Verification items for the finished model (mm, model axes). Face numbers are marked on the shaded views. A direction names the side the tool comes from. Round coordinates to 2 decimals unless told otherwise and drop trailing zeros. Write each loop counter-clockwise with the first axis right and the second up, starting at its lowest first coordinate (ties: lowest second). Pieces come first, ordered by that corner, then holes. Notation, with made-up numbers: M 38.5,28.25 L 50.5,28.25 A23 cw 50.5,51.25 Z; hole C -18,22.5 d4. An arc over 180 degrees is marked long. Answer in a Markdown table with one row per item. Add a question column.
1. Sectioned sample at A-A on z = 0. Record the cut outline in (x, y), plus the area to 3 significant figures.
2. Go/stop test with flat-tipped pins: pin 1 Ø2 at (x, y) = (1, 3) entering from -Z; pin 2 Ø3 at (x, y) = (7, 1) entering from -Z; pin 3 Ø2 at (x, y) = (-6.5, 5) entering from -Z. Record where each tip stops, or that it passes through.
3. Material ranges on probe 1 along X at (y, z) = (3, 0); probe 2 along Z at (x, y) = (1, 1.6); probe 3 along Y at (x, z) = (7, 5.75), recorded low to high.
4. Sectioned sample at B-B on y = 0.9. Record the cut outline in (x, z), plus the area to 3 significant figures.
5. Set-up check for the marked faces 1 and 2: record each of +Z, -Z, +X, -X, +Y, -Y from which the full face is reachable in a straight line by a thin tool's end or side.
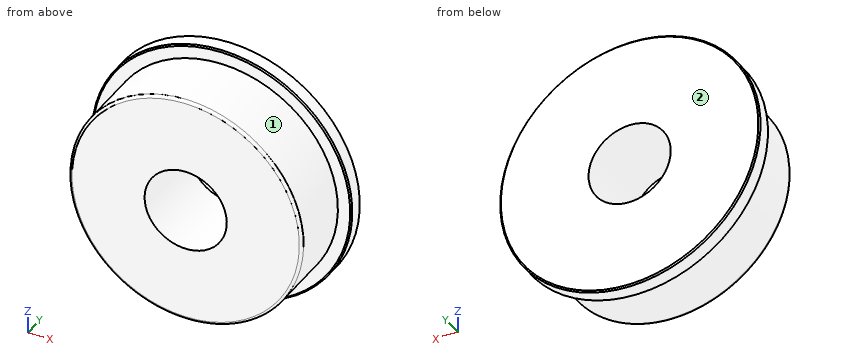
```python
from build123d import *

# Parameters (mm, degrees)
SKETCH_1_R      = 8.5
SKETCH_1_R_2    = 3
EXTRUDE_1_DEPTH = 6
EXTRUDE_START   = -1.2
SKETCH_2_R      = 9.5
SKETCH_2_R_2    = 3
EXTRUDE_2_DEPTH = 1.2
FILLET_1_R      = 0.2
CHAMFER_1_SIZE  = 0.1


with BuildPart() as part:
    # 草图1 → 凸台-拉伸1 (new body)
    with BuildSketch(Plane(origin=(0, 0, 0), x_dir=(1, 0, 0), z_dir=(0, 1, 0))):
        with Locations(Location((0, 0, 0), (0, 0, 270))):
            Circle(SKETCH_1_R)
        with Locations(Location((0, 0, 0), (0, 0, 270))):
            Circle(SKETCH_1_R_2, mode=Mode.SUBTRACT)
    extrude(amount=EXTRUDE_1_DEPTH)

    # 草图2 → 凸台-拉伸2 (add)
    with BuildSketch(Plane(origin=(0, 6, 0), x_dir=(1, 0, 0), z_dir=(0, 1, 0)).offset(EXTRUDE_START)):
        with Locations(Location((0, 0, 0), (0, 0, 270))):
            Circle(SKETCH_2_R)
        with Locations(Location((0, 0, 0), (0, 0, 270))):
            Circle(SKETCH_2_R_2, mode=Mode.SUBTRACT)
    extrude(amount=EXTRUDE_2_DEPTH)

    # 圆角1
    fillet_1_edges = [part.edges().sort_by_distance(p)[0] for p in [
        (0, 0, -8.5),
    ]]
    fillet(fillet_1_edges, radius=FILLET_1_R)

    # 倒角1
    chamfer_1_edges = [part.edges().sort_by_distance(p)[0] for p in [
        (0, 6, -9.5),
        (0, 4.8, -9.5),
    ]]
    chamfer(chamfer_1_edges, length=CHAMFER_1_SIZE)


solid = part.part
```
Geometry check:
| question | item | result |
|---|---|---|
| 1 | outline | M -9.5,4.9 L -9.4,4.8 L -8.5,4.8 L -8.5,0.2 A0.2 ccw -8.3,0 L -3,0 L -3,6 L -9.4,6 L -9.5,5.9 Z; M 3,0 L 8.3,0 A0.2 ccw 8.5,0.2 L 8.5,4.8 L 9.4,4.8 L 9.5,4.9 L 9.5,5.9 L 9.4,6 L 3,6 Z |
| 1 | area | 68.4 mm2 |
| 2 | pin 1 | stops at z = -8.5 |
| 2 | pin 2 | stops at z = -6.48 |
| 2 | pin 3 | stops at z = -7.75 |
| 3 | probe 1 | x = -8.5 to -3, 3 to 8.5 |
| 3 | probe 2 | z = -8.44 to -2.83, 2.83 to 8.44 |
| 3 | probe 3 | y = 4.8 to 6 |
| 4 | outline | C 0,0 d17; hole C 0,0 d6 |
| 4 | area | 199 mm2 |
| 5 | face 1 | -Y |
| 5 | face 2 | +Z, -Z, +X, -X, +Y |
